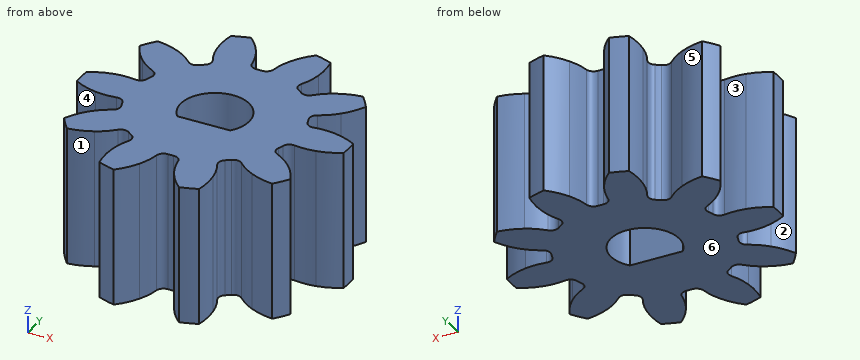
```python
from build123d import *

# Parameters (mm, degrees)
SKETCH1_R                = 5.887500036
BLANK_DISK_DEPTH         = 3.05
GEAR_TOOTH_CUT_DEPTH     = 11.321594513
GEAR_START               = -3.049999996
GEAR_TEETH_REVOLVE_DEPTH = 6.099999992
HUB_EXTRUDE_DEPTH        = 11.221001367


# Read off the part's stored shape, not the designer's step: GEAR TEETH REVOLVE
with BuildPart() as part:
    # Sketch1 → BLANK DISK (new, symmetric)
    with BuildSketch(Plane.XY):
        with Locations(Location((0, 0, 0), (0, 0, 180))):
            Circle(SKETCH1_R)
    extrude(amount=BLANK_DISK_DEPTH, both=True)

    # Sketch2 → GEAR TOOTH CUT (cut, through all)
    with BuildSketch(Plane.XY.offset(3.049999996)):
        with BuildLine():
            ThreePointArc((-4.985659759, -3.131429935), (-5.599345274, -1.819337566), (-5.874091808, -0.397117245))
            ThreePointArc((-5.874091808, -0.397117245), (-5.376423722, -0.629962338), (-4.845327653, -0.77077188))
            ThreePointArc((-4.845327653, -0.77077188), (-4.383437981, -0.811075473), (-3.921230969, -0.774590865))
            ThreePointArc((-3.921230969, -0.774590865), (-3.682257583, -0.823363871), (-3.535926696, -1.018490385))
            ThreePointArc((-3.535926696, -1.018490385), (-3.499590796, -1.137085978), (-3.459278416, -1.254389535))
            ThreePointArc((-3.459278416, -1.254389535), (-3.462970103, -1.498261339), (-3.627635579, -1.678184561))
            ThreePointArc((-3.627635579, -1.678184561), (-4.023014022, -1.920346358), (-4.373000758, -2.224444588))
            ThreePointArc((-4.373000758, -2.224444588), (-4.719900732, -2.650532337), (-4.985659759, -3.131429935))
        make_face()
    extrude(amount=-GEAR_TOOTH_CUT_DEPTH, mode=Mode.SUBTRACT)

    # GEAR TEETH REVOLVE outline → GEAR TEETH REVOLVE (cut)
    with BuildSketch(Plane.XY.offset(GEAR_START)):
        with BuildLine():
            ThreePointArc((-4.518820439, -3.773979135), (-3.460585694, -4.763087583), (-2.192875139, -5.463877313))
            ThreePointArc((-2.192875139, -5.463877313), (-2.260536085, -4.918613747), (-2.230336207, -4.369998828))
            ThreePointArc((-2.230336207, -4.369998828), (-2.125935444, -3.918261151), (-1.948406698, -3.489950524))
            ThreePointArc((-1.948406698, -3.489950524), (-1.920945745, -3.247601641), (-2.061303357, -3.048135288))
            ThreePointArc((-2.061303357, -3.048135288), (-2.162866059, -2.97692974), (-2.26197116, -2.902341595))
            ThreePointArc((-2.26197116, -2.902341595), (-2.495047822, -2.830492067), (-2.717049406, -2.931498908))
            ThreePointArc((-2.717049406, -2.931498908), (-3.069537619, -3.232694041), (-3.466904071, -3.471579687))
            ThreePointArc((-3.466904071, -3.471579687), (-3.979335588, -3.669832811), (-4.518820439, -3.773979135))
        make_face()
        with BuildLine():
            ThreePointArc((-1.437513252, -5.709309268), (0, -5.887500035), (1.437513252, -5.709309268))
            ThreePointArc((1.437513252, -5.709309268), (1.062276513, -5.307951883), (0.764240969, -4.846362048))
            ThreePointArc((0.764240969, -4.846362048), (0.583178216, -4.419533361), (0.475047319, -3.968674006))
            ThreePointArc((0.475047319, -3.968674006), (0.354814597, -3.756468498), (0.124019523, -3.677596963))
            ThreePointArc((0.124019523, -3.677596963), (0, -3.679687523), (-0.124019523, -3.677596963))
            ThreePointArc((-0.124019523, -3.677596963), (-0.354814597, -3.756468498), (-0.475047319, -3.968674006))
            ThreePointArc((-0.475047319, -3.968674006), (-0.583178216, -4.419533361), (-0.764240969, -4.846362048))
            ThreePointArc((-0.764240969, -4.846362048), (-1.062276513, -5.307951883), (-1.437513252, -5.709309268))
        make_face()
        with BuildLine():
            ThreePointArc((2.192875139, -5.463877313), (3.460585694, -4.763087583), (4.518820439, -3.773979135))
            ThreePointArc((4.518820439, -3.773979135), (3.979335588, -3.669832811), (3.466904071, -3.471579687))
            ThreePointArc((3.466904071, -3.471579687), (3.069537619, -3.232694041), (2.717049406, -2.931498908))
            ThreePointArc((2.717049406, -2.931498908), (2.495047822, -2.830492067), (2.26197116, -2.902341595))
            ThreePointArc((2.26197116, -2.902341595), (2.162866059, -2.97692974), (2.061303357, -3.048135288))
            ThreePointArc((2.061303357, -3.048135288), (1.920945745, -3.247601641), (1.948406698, -3.489950524))
            ThreePointArc((1.948406698, -3.489950524), (2.125935444, -3.918261151), (2.230336207, -4.369998828))
            ThreePointArc((2.230336207, -4.369998828), (2.260536085, -4.918613747), (2.192875139, -5.463877313))
        make_face()
        with BuildLine():
            ThreePointArc((4.985659759, -3.131429935), (5.599345274, -1.819337565), (5.874091808, -0.397117245))
            ThreePointArc((5.874091808, -0.397117245), (5.376423722, -0.629962338), (4.845327653, -0.77077188))
            ThreePointArc((4.845327653, -0.77077188), (4.383437981, -0.811075473), (3.921230969, -0.774590865))
            ThreePointArc((3.921230969, -0.774590865), (3.682257583, -0.823363871), (3.535926696, -1.018490385))
            ThreePointArc((3.535926696, -1.018490385), (3.499590796, -1.137085978), (3.459278416, -1.254389535))
            ThreePointArc((3.459278416, -1.254389535), (3.462970103, -1.498261338), (3.627635579, -1.678184561))
            ThreePointArc((3.627635579, -1.678184561), (4.023014022, -1.920346358), (4.373000758, -2.224444588))
            ThreePointArc((4.373000758, -2.224444588), (4.719900732, -2.650532336), (4.985659759, -3.131429935))
        make_face()
        with BuildLine():
            ThreePointArc((5.874091808, 0.397117245), (5.599345274, 1.819337566), (4.98565976, 3.131429935))
            ThreePointArc((4.98565976, 3.131429935), (4.719900732, 2.650532336), (4.373000758, 2.224444588))
            ThreePointArc((4.373000758, 2.224444588), (4.023014022, 1.920346358), (3.627635579, 1.678184561))
            ThreePointArc((3.627635579, 1.678184561), (3.462970103, 1.498261338), (3.459278416, 1.254389535))
            ThreePointArc((3.459278416, 1.254389535), (3.499590796, 1.137085978), (3.535926696, 1.018490385))
            ThreePointArc((3.535926696, 1.018490385), (3.682257583, 0.823363871), (3.921230969, 0.774590865))
            ThreePointArc((3.921230969, 0.774590865), (4.383437981, 0.811075473), (4.845327653, 0.77077188))
            ThreePointArc((4.845327653, 0.77077188), (5.376423722, 0.629962338), (5.874091808, 0.397117245))
        make_face()
        with BuildLine():
            ThreePointArc((4.51882044, 3.773979135), (3.460585695, 4.763087584), (2.192875139, 5.463877314))
            ThreePointArc((2.192875139, 5.463877314), (2.260536085, 4.918613747), (2.230336207, 4.369998828))
            ThreePointArc((2.230336207, 4.369998828), (2.125935444, 3.918261151), (1.948406698, 3.489950524))
            ThreePointArc((1.948406698, 3.489950524), (1.920945745, 3.247601641), (2.061303357, 3.048135288))
            ThreePointArc((2.061303357, 3.048135288), (2.162866059, 2.97692974), (2.26197116, 2.902341595))
            ThreePointArc((2.26197116, 2.902341595), (2.495047822, 2.830492067), (2.717049406, 2.931498908))
            ThreePointArc((2.717049406, 2.931498908), (3.069537619, 3.232694041), (3.466904071, 3.471579687))
            ThreePointArc((3.466904071, 3.471579687), (3.979335588, 3.669832811), (4.51882044, 3.773979135))
        make_face()
        with BuildLine():
            ThreePointArc((1.437513252, 5.709309269), (0, 5.887500037), (-1.437513252, 5.709309269))
            ThreePointArc((-1.437513252, 5.709309269), (-1.062276513, 5.307951883), (-0.764240969, 4.846362048))
            ThreePointArc((-0.764240969, 4.846362048), (-0.583178216, 4.419533361), (-0.475047319, 3.968674006))
            ThreePointArc((-0.475047319, 3.968674006), (-0.354814597, 3.756468498), (-0.124019523, 3.677596963))
            ThreePointArc((-0.124019523, 3.677596963), (0, 3.679687523), (0.124019523, 3.677596963))
            ThreePointArc((0.124019523, 3.677596963), (0.354814597, 3.756468498), (0.475047319, 3.968674006))
            ThreePointArc((0.475047319, 3.968674006), (0.583178216, 4.419533361), (0.764240969, 4.846362048))
            ThreePointArc((0.764240969, 4.846362048), (1.062276513, 5.307951883), (1.437513252, 5.709309269))
        make_face()
        with BuildLine():
            ThreePointArc((-2.192875139, 5.463877315), (-3.460585695, 4.763087584), (-4.51882044, 3.773979136))
            ThreePointArc((-4.51882044, 3.773979136), (-3.979335588, 3.669832811), (-3.466904071, 3.471579687))
            ThreePointArc((-3.466904071, 3.471579687), (-3.069537619, 3.232694041), (-2.717049406, 2.931498908))
            ThreePointArc((-2.717049406, 2.931498908), (-2.495047822, 2.830492067), (-2.26197116, 2.902341595))
            ThreePointArc((-2.26197116, 2.902341595), (-2.162866059, 2.97692974), (-2.061303357, 3.048135288))
            ThreePointArc((-2.061303357, 3.048135288), (-1.920945745, 3.247601641), (-1.948406698, 3.489950524))
            ThreePointArc((-1.948406698, 3.489950524), (-2.125935444, 3.918261151), (-2.230336207, 4.369998828))
            ThreePointArc((-2.230336207, 4.369998828), (-2.260536085, 4.918613747), (-2.192875139, 5.463877315))
        make_face()
        with BuildLine():
            ThreePointArc((-3.535926696, 1.018490385), (-3.499590796, 1.137085978), (-3.459278416, 1.254389535))
            ThreePointArc((-3.459278416, 1.254389535), (-3.462970103, 1.498261338), (-3.627635579, 1.678184561))
            ThreePointArc((-3.627635579, 1.678184561), (-4.023014022, 1.920346358), (-4.373000758, 2.224444588))
            ThreePointArc((-4.373000758, 2.224444588), (-4.719900732, 2.650532336), (-4.985659759, 3.131429935))
            ThreePointArc((-4.985659759, 3.131429935), (-5.599345274, 1.819337566), (-5.874091808, 0.397117245))
            ThreePointArc((-5.874091808, 0.397117245), (-5.376423722, 0.629962338), (-4.845327653, 0.77077188))
            ThreePointArc((-4.845327653, 0.77077188), (-4.383437981, 0.811075473), (-3.921230969, 0.774590865))
            ThreePointArc((-3.921230969, 0.774590865), (-3.682257583, 0.823363871), (-3.535926696, 1.018490385))
        make_face()
    extrude(amount=GEAR_TEETH_REVOLVE_DEPTH, mode=Mode.SUBTRACT)

    # Sketch3 → HUB EXTRUDE (cut, through all)
    with BuildSketch(Plane.XY.offset(3.049999996)):
        with BuildLine():
            Line((-1.169092, -0.9398), (1.169092, -0.9398))
            ThreePointArc((1.169092, -0.9398), (0, 1.500000048), (-1.169092, -0.9398))
        make_face()
    extrude(amount=-HUB_EXTRUDE_DEPTH, mode=Mode.SUBTRACT)


solid = part.part
```
CAD build for the part. Positions are in the model's coordinates, mm. Face numbers are marked on the shaded views. A direction names the side the tool comes from. Round coordinates to 2 decimals unless told otherwise and drop trailing zeros. Loops run counter-clockwise (first coordinate to the right, second up) from the corner with the lowest first, then second, coordinate; pieces in that order, holes last. Notation, with made-up numbers: (41, 69.5) - (66, 69.5) arc R4 cw to (66, 76.5) - close; hole circle Ø3 at (81, 69). An arc over 180 degrees is marked (long way). Return JSON: item names as keys, results as strings. Group by question number.
Q1. Band-saw the part on A-A on y = 0. Give the cut face in (x, z), plus the area to 3 significant figures.
Q2. Tool access for the marked faces 1, 2 and 3: list every direction of +Z, -Z, +X, -X, +Y, -Y with a clear straight run to the whole face (end or side of a thin tool).
Q3. Band-saw the part on B-B on y = -2. Give the cut face in (x, z), plus the area to 3 significant figures.
Q4. Drill centre lines: line 1 along X through (y, z) = (0, -0.5); line 2 along Y through (x, z) = (-4.25, 2); line 3 along X through (y, z) = (-3.5, 2.5). Where is each one in solid material? Low to high. Write a range as [from, to].
Q5. Flat gauge pin, fed straight in: pin 1 Ø0.7 at (x, z) = (0.5, 1.5) entering from +Y. Where does the tip first touch, or does it go through?
Q6. Two-plate mould, pull along X, no slides. Class the marked faces 4, 5 and 6: +X half, -X half, draft (parallel to the pull), parting line (faces both ways), or undercut.
Solutions:
{
 "1": {"outline": "(-5.89, -3.05) - (-1.5, -3.05) - (-1.5, 3.05) - (-5.89, 3.05) - close; (1.5, -3.05) - (5.89, -3.05) - (5.89, 3.05) - (1.5, 3.05) - close", "area": "53.5 mm^2"},
 "2": {"face 1": "+Z, -Z, -Y", "face 2": "+Z, -Z, -X", "face 3": "+Z, -Z"},
 "3": {"outline": "(-4.13, -3.05) - (4.13, -3.05) - (4.13, 3.05) - (-4.13, 3.05) - close", "area": "50.3 mm^2"},
 "4": {"line 1": "x = [-5.89, -1.5], [1.5, 5.89]", "line 2": "y = [-3.73, -2.11], [-0.81, 0.81], [2.11, 3.73]", "line 3": "x = [-4.73, -3.53], [-1.95, 1.95], [3.53, 4.73]"},
 "5": {"pin 1": "stops at y = 5"},
 "6": {"face 4": "-X half", "face 5": "undercut", "face 6": "draft"}
}
